Could you check a few things on this model? Use its own coordinates, in mm. Face numbers are marked on the shaded views. A direction names the side the tool comes from. Round coordinates to 2 decimals unless told otherwise and drop trailing zeros. Loops run counter-clockwise (first coordinate to the right, second up) from the corner with the lowest first, then second, coordinate; pieces in that order, holes last. Notation, with made-up numbers: (59.25, 13.5) - (118.25, 13.5) arc R22 ccw to (118.25, 45.5) - close; hole circle Ø6 at (37.5, 34.25). An arc over 180 degrees is marked (long way). Put each result on its own line as item: value. Start each with the question number.
from build123d import *

# Parameters (mm, degrees)
F0_R     = 9.144
F1_DEPTH = 9.525
F2_R     = 6.35
F3_DEPTH = 6.35
F4_W     = 15.875
F4_H     = 6.35
F5_DEPTH = 6.35
F6_R     = 1.5875
F7_DEPTH = 3.175


with BuildPart() as f1:
    # F0 (on Top) → F1 (new body)
    with BuildSketch(Plane.XY):
        Circle(F0_R)
    extrude(amount=F1_DEPTH)

    # F2 (on face) → F3 (cut)
    with BuildSketch(Plane.XY.offset(9.525)):
        Circle(F2_R)
    extrude(amount=-F3_DEPTH, mode=Mode.SUBTRACT)

    # F4 (on face) → F5 (join)
    with BuildSketch(Plane(origin=(0, 0, 0), x_dir=(1, 0, 0), z_dir=(0, 0, -1))):
        Rectangle(F4_W, F4_H)
    extrude(amount=F5_DEPTH)

    # F6 (on Front) → F7 (join, symmetric)
    with BuildSketch(Plane.XZ):
        with BuildLine():
            Line((7.9375, -6.35), (-7.9375, -6.35))
            ThreePointArc((-7.9375, -6.35), (0, -14.2875), (7.9375, -6.35))
        make_face()
        with Locations((0, -10.31875)):
            Circle(F6_R, mode=Mode.SUBTRACT)
    extrude(amount=F7_DEPTH, both=True)


solid = f1.part
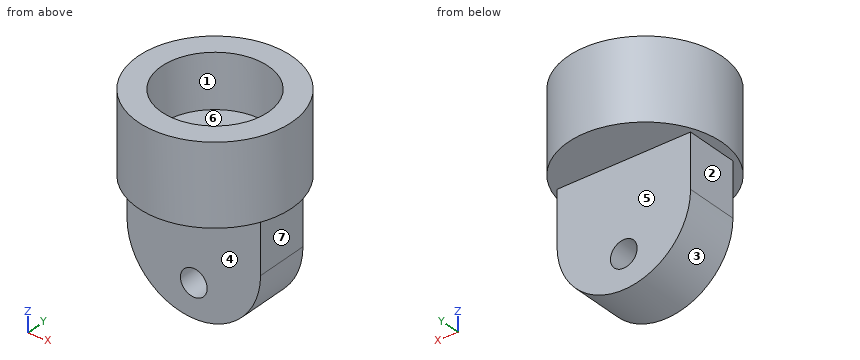
Item 1: Suppose I cut it at B-B, the plane z = -9.5. List the corners of the cut face in (x, y) for me (3 decimals), then the cut area to 3 significant figures.
Item 2: On a 3-axis mill with a long thin cutter (end or side, diameter ignored), from which of +Z, -Z, +X, -X, +Y, -Y can I reach the whole of each face in a straight line? I mean the marked faces 4, 5, 6 and 7. Say none if no direction works.
Item 3: I need wall thicknesses on line 1 (Y direction, x = 0, z = 7.75); line 2 (Z direction, x = 0, y = 1) (1 decimal); line 3 (Y direction, x = 2.75, z = -2) (3 decimals). Which ranges of each line are inside material? Lowest first, please. Write a range as from..to.
Item 4: Suppose I cut it at D-D, the plane x = -5. List the corners of the cut face in (y, z) for me (3 decimals), then the cut area to 3 significant figures.
Item 5: Thinking about a two-plate mould opening in X: for the marked faces 1, 2 and 3, which applies, released by +X, released by -X, zero draft, split by the parting line, or undercut?
Item 6: Will these pins go through, and if not, where does the flat tip stop? P1, Ø1, axis at y = 1.5, z = 0.5, coming from the -X side; P2, Ø3, axis at y = 1.5, z = -3, coming from the -X side; P3, Ø1.5, axis at x = 5, y = -1.5, coming from the +Z side (3 decimals).
Numbers:
1. outline: (-7.286, -3.175) - (-1.36, -3.175) - (-1.36, 3.175) - (-7.286, 3.175) - close; (1.36, -3.175) - (7.286, -3.175) - (7.286, 3.175) - (1.36, 3.175) - close
1. area: 75.3 mm^2
2. face 4: -Z, +X, -X, -Y
2. face 5: -Z, +X, -X, +Y
2. face 6: +Z
2. face 7: -Z, +X, +Y, -Y
3. line 1: -9.14..-6.35, 6.35..9.14
3. line 2: -14.3..-11.9, -8.7..3.2
3. line 3: -3.175..3.175
4. outline: (-7.656, 0) - (-3.175, 0) - (-3.175, -12.515) - (3.175, -12.515) - (3.175, 0) - (7.656, 0) - (7.656, 9.525) - (3.914, 9.525) - (3.914, 3.175) - (-3.914, 3.175) - (-3.914, 9.525) - (-7.656, 9.525) - close
4. area: 176 mm^2
5. face 1: undercut
5. face 2: released by -X
5. face 3: split by the parting line
6. P1: x = -9.09
6. P2: x = -7.94
6. P3: z = 3.175
